Design review of the part built by this model. Coordinates are the model's own, in mm. A direction names the side the tool comes from. Give positions to 0.01 mm unless a question says otherwise; leave off trailing zeros. Order: outer loops, then holes, each group sorted by start corner. A loop starts at its lowest first (then second) coordinate and runs counter-clockwise, first axis right, second up. Notation, with made-up numbers: M 19.25,86.25 L 34.25,86.25 A14 cw 34.25,99.25 Z; hole C 18.5,-8.5 d3. An arc over 180 degrees is marked long. Answer as a JSON object with one key per item and string values.
from build123d import *

# Parameters (mm, degrees)
EXTRUDE_1_DEPTH        = 8
HOLE_WIZARD_M2_1_D     = 2.459
HOLE_WIZARD_M2_1_DEPTH = 13.499999938
HOLE_WIZARD_M2_2_D     = 2.459
HOLE_WIZARD_3_0_3_1_D  = 3
CHAMFER_1_SIZE         = 0.2705


with BuildPart() as part:
    # 草图1 → 凸台-拉伸1 (new body)
    with BuildSketch(Plane(origin=(0, 4, 0), x_dir=(1, 0, 0), z_dir=(0, 1, 0))):
        with BuildLine():
            Line((-2.499999938, 2.449489682), (-2.499999938, -28.00000006))
            ThreePointArc((-2.499999938, -28.00000006), (-2.267766887, -28.267767018), (-1.999999928, -28.500000068))
            Line((-1.999999928, -28.500000068), (2.000000062, -28.500000068))
            ThreePointArc((2.000000062, -28.500000068), (2.267767019, -28.267767016), (2.500000069, -28.000000058))
            Line((2.500000069, -28.000000058), (2.500000069, -10.7))
            Line((2.500000069, -10.7), (3.21, -10.7))
            ThreePointArc((3.21, -10.7), (3.393052661, -10.517652269), (3.616779061, -10.388402631))
            ThreePointArc((3.616779061, -10.388402631), (9.876142021, -4.843740163), (10.428326836, 3.499999914))
            Line((10.428326836, 3.499999914), (0, 3.499999914))
            ThreePointArc((0, 3.499999914), (-1.355873467, 3.226702114), (-2.499999938, 2.449489682))
        make_face()
    extrude(amount=-EXTRUDE_1_DEPTH)

    # M2 间隙孔1
    with Locations(Plane.ZY.offset(2.499999938)):
        with Locations((17.5, 0)):
            Hole(HOLE_WIZARD_M2_1_D / 2, depth=HOLE_WIZARD_M2_1_DEPTH)

    # M2 间隙孔2 (through all)
    with Locations(Plane(origin=(2.500000069, 0, 0), x_dir=(0, 0, -1), z_dir=(1, 0, 0))):
        with Locations((-24.500000001, 0)):
            Hole(HOLE_WIZARD_M2_2_D / 2)

    # Ø3.0 (3) 直径孔1 (through all)
    with Locations(Plane(origin=(0, 4, 0), x_dir=(1, 0, 0), z_dir=(0, 1, 0))):
        with Locations((0, 0)):
            Hole(HOLE_WIZARD_3_0_3_1_D / 2)

    # 倒角1
    chamfer_1_edges = [part.edges().sort_by_distance(p)[0] for p in [
        (2.500000069, 0, 18.7295),
        (-2.499999938, 0, 18.7295),
        (2.500000069, 0, 23.270500001),
        (-2.499999938, 0, 23.270500001),
    ]]
    chamfer(chamfer_1_edges, length=CHAMFER_1_SIZE)


solid = part.part
(1) We need section D-D (y = 2.5). Write out the cut boundary in (x, z).
Checked values:
{"outline": "M -2.5,-2.45 A3.5 ccw 0,-3.5 L 10.43,-3.5 A11 ccw 3.62,10.39 A1 cw 3.21,10.7 L 2.5,10.7 L 2.5,28 A2.5 ccw 2,28.5 L -2,28.5 A2.5 ccw -2.5,28 Z; hole C 0,0 d3"}
(2) To check wall thickness, follow L1, parallel to Y at x = -0.55, z = 17.5; L2, parallel to Z at x = 0, y = -0.5; L3, parallel to Z at x = 0, y = -1.75. State the ranges of each line that lie inside material, in increasing order. Write a range as from..to.
Checked values:
{"L1": "y = -4..-1.23, 1.23..4", "L2": "z = -3.5..-1.5, 1.5..16.38, 18.62..23.38, 25.62..28.5", "L3": "z = -3.5..-1.5, 1.5..28.5"}
(3) We need section B-B (z = 17.5). Write out the cut boundary in (x, y).
Checked values:
{"outline": "M -2.5,-4 L 2.5,-4 L 2.5,-1.5 L 2.23,-1.23 L -2.23,-1.23 L -2.5,-1.5 Z; M -2.5,1.5 L -2.23,1.23 L 2.23,1.23 L 2.5,1.5 L 2.5,4 L -2.5,4 Z"}
(4) Insertion check: pin 1 (4 mm diameter, centred on y = 0, z = 24.5, fed in from +X); pin 2 (0.6 mm diameter, centred on x = 3, y = -1.5, fed in from +Z). Each pin has a flat end and moves straight along its axis. Give the tip position at first contact, or say it passes through.
Checked values:
{"pin 1": "stops at x = 2.5", "pin 2": "stops at z = 10.7"}
(5) We need section A-A (y = 0). Write out the cut boundary in (x, z), plus the area to 3 significant figures.
Checked values:
{"outline": "M -2.5,-2.45 A3.5 ccw 0,-3.5 L 10.43,-3.5 A11 ccw 3.62,10.39 A1 cw 3.21,10.7 L 2.5,10.7 L 2.5,16 L 2.23,16.27 L -2.23,16.27 L -2.5,16 Z; M -2.5,19 L -2.23,18.73 L 2.23,18.73 L 2.5,19 L 2.5,23 L 2.23,23.27 L -2.23,23.27 L -2.5,23 Z; M -2.5,26 L -2.23,25.73 L 2.23,25.73 L 2.5,26 L 2.5,28 A2.5 ccw 2,28.5 L -2,28.5 A2.5 ccw -2.5,28 Z; hole C 0,0 d3", "area": "224 mm^2"}
(6) We need section C-C (x = -0.75). Write out the cut boundary in (y, z).
Checked values:
{"outline": "M -4,-3.42 L 4,-3.42 L 4,-1.3 L -4,-1.3 Z; M -4,1.3 L 4,1.3 L 4,28.5 L -4,28.5 Z; hole C 0,17.5 d2.46; hole C 0,24.5 d2.46"}
(7) Draft analysis for pull direction Z (two halves, no side actions). For faces 3 (the flat face through (0, 0, 28.5)), 4 (the flat face through (3, 4, 9)), 5 (the cylindrical face through (-0.031, -0.471, 25.636)), state which applies: +Z half, -Z half, draft (parallel to the pull), parting line (faces both ways), or undercut.
Checked values:
{"face 3": "+Z half", "face 4": "draft", "face 5": "undercut"}
(8) Tool access review of faces 1 (the flat face through (2.5, 0.1, 19.5)), 2 (the flat face through (5, 0, -3.5)): name each direction out of +Z, -Z, +X, -X, +Y, -Y from which nothing blocks a thin tool from reaching the whole face with its end or side.
Checked values:
{"face 1": "+Z, +X, +Y, -Y", "face 2": "-Z, +X, -X, +Y, -Y"}
